Geometry: final body of the model. Coordinates: model frame, mm. Face numbers are marked on the shaded views. A direction names the side the tool comes from. Give positions to 0.01 mm unless a question says otherwise; leave off trailing zeros. Write each loop counter-clockwise with the first axis right and the second up, starting at its lowest first coordinate (ties: lowest second). Pieces come first, ordered by that corner, then holes. Notation, with made-up numbers: (71.25, 28) - (75.25, 28) arc R16 cw to (75.25, 43) - close; hole circle Ø4 at (-5, -10). An arc over 180 degrees is marked (long way). Use CSV: the item, a comma, the result in double quotes. Start each with the question number.
(1) Line query: probe 1 along Y at (x, z) = (-14, 9.5); probe 2 along Z at (x, y) = (-5.5, 1); probe 3 along X at (y, z) = (43, -4). Output: solid intervals per line, ascending. Write a range as [from, to].
(2) Draft query along Y for the marked faces 3, 4 and 5. Return one class per face: released by +Y, released by -Y, zero draft, split by the parting line, or undercut.
(3) Section A-A on y = 42.5. Output: boundary loops of the cut face in (x, z), and give its area (3 significant figures).
(4) First-contact query: pin 1 Ø6 at (y, z) = (41, -10) entering from -X; pin 2 Ø8 at (x, z) = (-19.5, 6.5) entering from -Y; pin 3 Ø2 at (y, z) = (25, -8) entering from -X. Flat tips, straight axial feed; report the tip coordinate or a pass-through.
(5) Section B-B on x = 10. Output: boundary loops of the cut face in (y, z).
(6) Reachability of the marked faces 1 and 2 from +Z, -Z, +X, -X, +Y, -Y: full face, straight path, thin tool, end or side. Return the list, or none.
Autodesk Inventor part; units mm, degrees
ref_plane "Work Plane1" through (0, 14.5, 0) normal (0, 1, 0) x (-1, 0, 0)
ref_plane "Work Plane3" through (-19.799, -5.299, 14.5) normal (-0.7071068, -0.7071068, 0) x (0, 0, -1)
ref_plane "YZ Plane" through (0, 0, 0) normal (1, 0, 0) x (0, 1, 0)
sketch "Sketch1" plane through (0, 0, 0) normal (0, 0, 1) x (1, 0, 0)
  line L0 (0, 0) -> (0, 14.5) construction
  line L1 (0, 0) -> (31.6, 0) construction
  line L2 (31.6, 0) -> (31.6, 14) construction
  line L3 (0, 12.4997) -> (31.6, 11.9997)
  line L4 (0, 12.4997) -> (0, 14.5)
  line L5 (31.6, 14) -> (31.6, 11.9997)
  line L6 (29.6, 0) -> (29.6, 13.2) construction
  line L7 (29.6, 13.2) -> (29.6132, 14.0314)
  line L8 (29.6, 13.2) -> (26.4004, 13.2506)
  line L9 (26.4004, 13.2506) -> (26.4136, 14.0821)
  line L10 (31.6, 14) -> (29.6132, 14.0314)
  line L11 (26.4136, 14.0821) -> (0, 14.5)
  dimension "d0" = 14.5
  dimension "d1" = 31.6
  dimension "d2" = 14
  dimension "d4" = 13.2
  dimension "d5" = 2
  dimension "d6" = 3.2
  dimension "d22" = 2
revolve "Revolution1" add sketch "Sketch1" angle 360 about axis through (0, 0, 0) along (1, 0, 0)
ref_plane "Work Plane1" through (0, 14.5, 0) normal (0, 1, 0) x (-1, 0, 0)
sketch "Sketch2" plane through (0, 14.5, 0) normal (0, 1, 0) x (-1, 0, 0)
  line L0 (0, 14.5) -> (0, -14.5) construction
  line L1 (0, 14.5) -> (0, -14.5) construction
  point P0 (0, 0)
sketch "Sketch3" plane through (0, 0, 0) normal (-1, 0, 0) x (0, 0, 1)
  circle A0 centre (0, 0) radius 14.5
  circle A1 centre (0, 0) radius 12.4997
revolve "Revolution2" add sketch "Sketch3" angle 90 about axis through (0, 14.5, 14.5) along (0, 0, -1)
sketch "Sketch4" plane through (0, 0, 0) normal (0, 0, 1) x (1, 0, 0)
  line L0 (0, 14.5) -> (-29, 14.5) construction
  line L1 (-14.5, 14.5) -> (0, 14.5) construction
  line L2 (0, 14.5) -> (26.4136, 14.0821) construction
  line L3 (-14.5, 14.5) -> (-14.5, 29.5) construction
  line L4 (-14.5, 29.5) -> (-3.25, 29.5) construction
  line L5 (-3.25, 29.5) -> (0, 14.5)
  line L6 (-14.5, 29.5) -> (-14.5, 54.5) construction
  line L7 (-14.5, 54.5) -> (-3.5, 54.5) construction
  line L8 (-3.5, 54.5) -> (-3.25, 29.5)
  line L9 (-3.5, 54.5) -> (-4.7, 54.5)
  line L10 (-4.7, 54.5) -> (-4.45, 29.5)
  line L11 (-4.45, 29.5) -> (-2.0003, 14.5)
  line L12 (-2.0003, 14.5) -> (0, 14.5)
  line L13 (-26.9997, 14.5) -> (-2.0003, 14.5)
  point P0 (0, 0)
  dimension "d10" = 15
  dimension "d11" = 11.25
  dimension "d12" = 25
  dimension "d13" = 11
  dimension "d14" = 1.2
  dimension "d15" = 1.2
revolve "Revolution3" add sketch "Sketch4" angle 360 about axis through (-14.5, 29.5, 0) along (0, 1, 0)
ref_plane "Work Plane3" through (-19.799, -5.299, 14.5) normal (-0.7071068, -0.7071068, 0) x (0, 0, -1)
ref_plane "Work Plane2" through (0, 14.5, 14.5) normal (-0.7071068, -0.7071068, 0) x (0, 0, -1)
sketch "Sketch5" plane through (-19.799, -5.299, 14.5) normal (-0.7071068, -0.7071068, 0) x (0, 0, -1)
  circle A0 centre (14.5, 0) radius 14.5
  point P0 (14.5, 10.253)
extrude "Extrusion1" cut sketch "Sketch5" along normal blind 10
sketch "Sketch6" plane through (-19.799, -5.299, 14.5) normal (-0.7071068, -0.7071068, 0) x (-0.7071068, 0.7071068, 0)
  ellipse E0 centre (-10.253, 14.5) end of major axis (-10.253, 29) minor radius 10.253
  circle A0 centre (0, 14.5) radius 12.5
  dimension "d23" = 25
extrude "Extrusion2" add sketch "Sketch6" against normal up to next contours A0 E0 | E0 A0 picked at (-4.1364, 16.63) picked at (3.9536, 16.6096)
sketch "Sketch7" plane through (0, 0, 0) normal (0, 0, 1) x (1, 0, 0)
  line L0 (0, 0) -> (0, 15) construction
  line L1 (0, -14.5) -> (0, 14.5)
  line L2 (0, 14.5) -> (0, 15)
  line L3 (31.6, -14) -> (31.6, 14)
  line L4 (0, 15) -> (31.6, 14)
  line L5 (26.4136, -14.0821) -> (26.4136, 14.0821)
  line L6 (26.4136, 14.0821) -> (26.4162, 14.164)
  line L7 (29.6132, -14.0314) -> (29.6132, 14.0314)
  line L8 (29.6132, 14.0314) -> (29.6141, 14.0628)
  line L9 (0, 14.5) -> (26.4136, 14.0821)
  line L10 (29.6132, 14.0314) -> (31.6, 14)
  line L11 (31.6, -11.9997) -> (31.6, 11.9997)
  line L12 (31.6, 0) -> (0, 0)
  dimension "d26" = 15
revolve "Revolution4" add sketch "Sketch7" angle 360 about axis through (31.6, 0, 0) along (-1, 0, 0) contours L2 L4 L6 L9 | L8 L4 L10
properties part number "90DegreeV3"
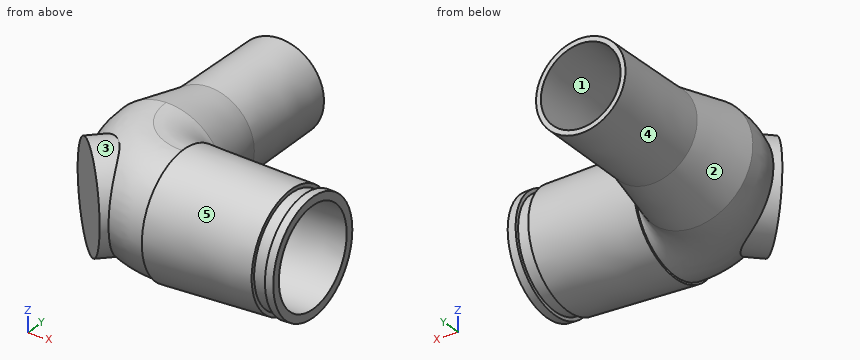
Check values:
1,probe 1,"y = [-10.99, -3.27]"
1,probe 2,"z = [-14.5, -12.5], [12.5, 14.5]"
1,probe 3,"x = [-24.87, -23.57], [-5.43, -4.13]"
2,face 3,"undercut"
2,face 4,"released by +Y"
2,face 5,"split by the parting line"
3,outline,"circle Ø22.24 at (-14.5, 0); hole circle Ø19.84 at (-14.5, 0)"
3,area,"79.3 mm²"
4,pin 1,"stops at x = -23.16"
4,pin 2,"stops at y = -9.6"
4,pin 3,"stops at x = -24.57"
5,outline,"circle Ø29.37 at (0, 0); hole circle Ø24.68 at (0, 0)"
6,face 1,"none"
6,face 2,"+Y"
